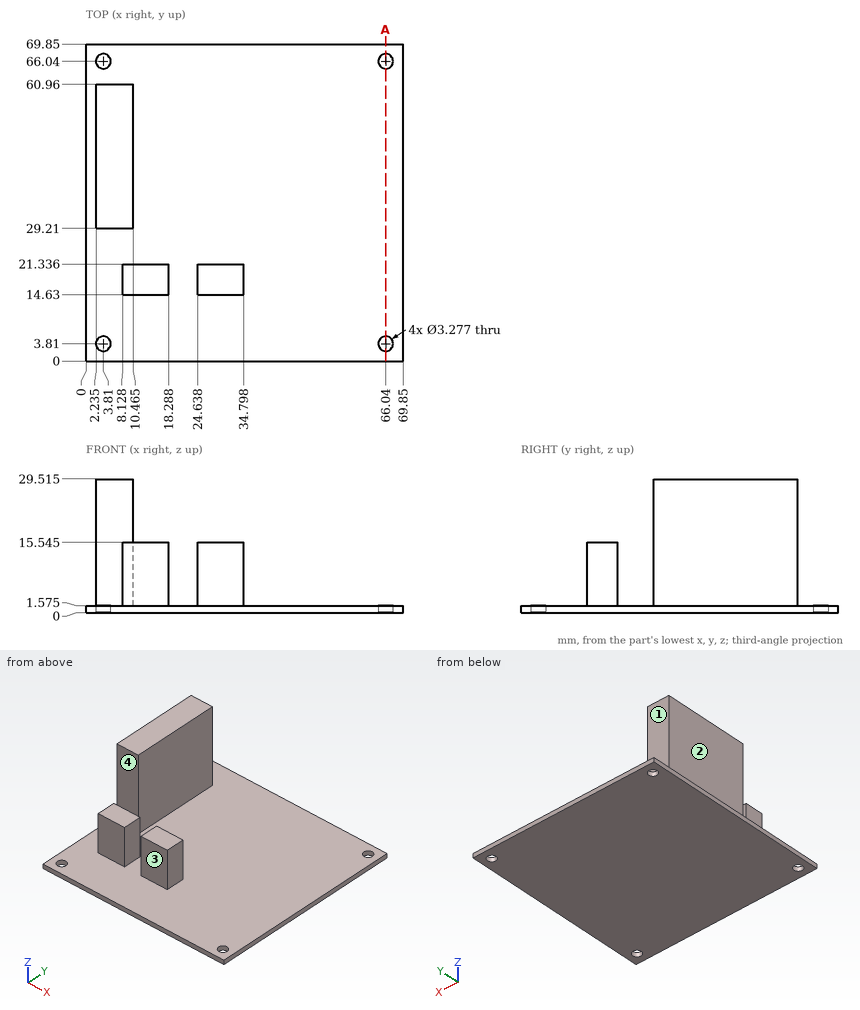
Geometry check sheet. Reference: drawing and pictorial views, mm from the part's lowest x, y, z. A direction names the side the tool comes from. Round coordinates to 2 decimals unless told otherwise and drop trailing zeros. Answer as CSV lines item,"result".
1) Tool access check on the marked faces 1, 2, 3 and 4. Record the directions out of +Z, -Z, +X, -X, +Y, -Y that give a thin tool (end or side, any length) a straight path to the whole face; none if there is none.
Entries:
face 1,"+Z, +X, -X, +Y"
face 2,"+Z, -X, +Y, -Y"
face 3,"+Z, +X, -X, -Y"
face 4,"+Z, +X, -X"
2) Sectioned sample at A-A on x = 66.04. Give the number of separate pieces and of enclosed holes in the cut face.
Entries:
separate pieces,"3"
enclosed holes,"0"
3) Gauge pin test, flat ends, axial feed: pin 1 Ø2 at (x, y) = (66.04, 3.81) entering from -Z; pin 2 Ø6 at (x, y) = (21, 39) entering from +Z (1 decimal); pin 3 Ø9 at (x, z) = (5.5, 13.5) entering from -Y; pin 4 Ø3.5 at (x, y) = (29.5, 16.5) entering from +Z (1 decimal). Record the tip position at first contact, or that the pin passes through.
Entries:
pin 1,"through"
pin 2,"z = 1.6"
pin 3,"y = 14.63"
pin 4,"z = 15.5"
4) Thickness scan on probe 1 along Y at (x, z) = (3.81, 1.15); probe 2 along Z at (x, y) = (57, 38.5) (1 decimal). Record the ranges inside material, lowest first. Write a range as [from, to].
Entries:
probe 1,"[0, 2.17], [5.45, 64.4], [67.68, 69.85]"
probe 2,"[0, 1.6]"
